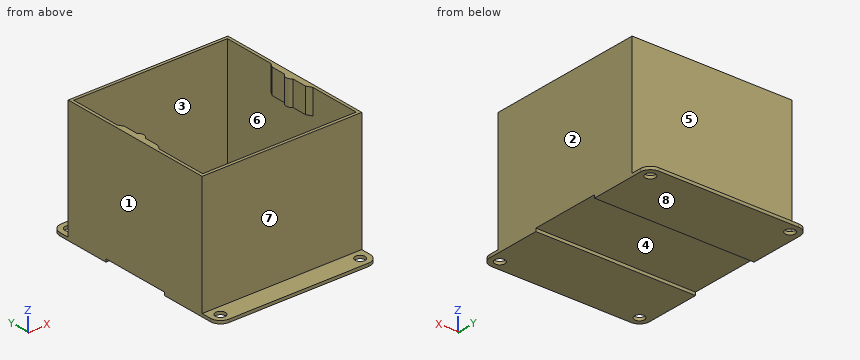
```python
from build123d import *

# Parameters (mm, degrees)
F0_W     = 101.6
F0_H     = 101.6
F1_DEPTH = 76.2
F2_W     = 97.80524
F2_H     = 97.80524
F3_DEPTH = 74.30262
F5_DEPTH = 15.875
F6_R     = 3.175
F7_DEPTH = 1.89738


with BuildPart() as f1:
    # F0 (on Top) → F1 (new body)
    with BuildSketch(Plane.XY):
        Rectangle(F0_W, F0_H)
    extrude(amount=F1_DEPTH)

    # F2 (on face) → F3 (cut)
    with BuildSketch(Plane.XY.offset(76.2)):
        Rectangle(F2_W, F2_H)
    extrude(amount=-F3_DEPTH, mode=Mode.SUBTRACT)

    # F4 (on face) → F5 (join)
    with BuildSketch(Plane.XY.offset(76.2)):
        with BuildLine():
            Line((-47.00524, 12.7), (-48.90262, 15.986359))
            Line((-48.90262, 15.986359), (-48.90262, -15.986359))
            Line((-48.90262, -15.986359), (-47.00524, -12.7))
            Line((-47.00524, -12.7), (-47.00524, -3.175))
            ThreePointArc((-47.00524, -3.175), (-45.301297, 0), (-47.00524, 3.175))
            Line((-47.00524, 3.175), (-47.00524, 12.7))
        make_face()
        with BuildLine():
            Line((48.90262, -15.986359), (48.90262, 15.986359))
            Line((48.90262, 15.986359), (47.00524, 12.7))
            Line((47.00524, 12.7), (47.00524, 3.175))
            ThreePointArc((47.00524, 3.175), (45.301297, 0), (47.00524, -3.175))
            Line((47.00524, -3.175), (47.00524, -12.7))
            Line((47.00524, -12.7), (48.90262, -15.986359))
        make_face()
    extrude(amount=-F5_DEPTH)

    # F6 (on face) → F7 (join)
    with BuildSketch(Plane(origin=(0, 0, 0), x_dir=(1, 0, 0), z_dir=(0, 0, -1))):
        with BuildLine():
            Line((-50.8, 57.15), (-50.8, 22.225))
            Line((-50.8, 22.225), (50.8, 22.225))
            Line((50.8, 22.225), (50.8, 57.15))
            ThreePointArc((50.8, 57.15), (48.940128, 61.640128), (44.45, 63.5))
            Line((44.45, 63.5), (-44.45, 63.5))
            ThreePointArc((-44.45, 63.5), (-48.940128, 61.640128), (-50.8, 57.15))
        make_face()
        with Locations((-44.45, 57.15)):
            Circle(F6_R, mode=Mode.SUBTRACT)
        with Locations((44.45, 57.15)):
            Circle(F6_R, mode=Mode.SUBTRACT)
        with BuildLine():
            Line((50.8, -22.225), (-50.8, -22.225))
            Line((-50.8, -22.225), (-50.8, -57.15))
            ThreePointArc((-50.8, -57.15), (-48.940128, -61.640128), (-44.45, -63.5))
            Line((-44.45, -63.5), (44.45, -63.5))
            ThreePointArc((44.45, -63.5), (48.940128, -61.640128), (50.8, -57.15))
            Line((50.8, -57.15), (50.8, -22.225))
        make_face()
        with Locations((-44.45, -57.15)):
            Circle(F6_R, mode=Mode.SUBTRACT)
        with Locations((44.45, -57.15)):
            Circle(F6_R, mode=Mode.SUBTRACT)
    extrude(amount=F7_DEPTH)


solid = f1.part
```
Read the model definition and answer for the solid it produces. Units are mm, in the model's axes. Face numbers are marked on the shaded views. A direction names the side the tool comes from. Coordinates: 2 decimals unless noted, no trailing zeros. Loops run counter-clockwise (first coordinate to the right, second up) from the corner with the lowest first, then second, coordinate; pieces in that order, holes last. Notation, with made-up numbers: (1.25, 67) -> (21.25, 67) arc R23 ccw to (21.25, 101) -> close; hole circle Ø1 at (-12, 37). An arc over 180 degrees is marked (long way). Return JSON: item names as keys, results as strings.
Item 1: For a pull along X with two mould halves and no side action, classify the marked faces 1, 2, 3 and 4 as +X half, -X half, draft (parallel to the pull), parting line (faces both ways), or undercut.
Answers:
{"face 1": "-X half", "face 2": "+X half", "face 3": "undercut", "face 4": "draft"}
Item 2: Find section C-C (x = 18). Determine the outline of the cut face in (y, z) (3 decimals), plus the area to 3 significant figures.
Answers:
{"outline": "(-63.5, -1.897) -> (-22.225, -1.897) -> (-22.225, 0) -> (22.225, 0) -> (22.225, -1.897) -> (63.5, -1.897) -> (63.5, 0) -> (50.8, 0) -> (50.8, 76.2) -> (48.903, 76.2) -> (48.903, 1.897) -> (-48.903, 1.897) -> (-48.903, 76.2) -> (-50.8, 76.2) -> (-50.8, 0) -> (-63.5, 0) -> close", "area": "631 mm2"}
Item 3: Find section A-A (z = 67). Determine the outline of the cut face in (x, y) (3 decimals), plus the area to 3 significant figures.
Answers:
{"outline": "(-50.8, -50.8) -> (50.8, -50.8) -> (50.8, 50.8) -> (-50.8, 50.8) -> close; hole (-48.903, -48.903) -> (48.903, -48.903) -> (48.903, -15.986) -> (47.005, -12.7) -> (47.005, -3.175) arc R3.81 cw to (47.005, 3.175) -> (47.005, 12.7) -> (48.903, 15.986) -> (48.903, 48.903) -> (-48.903, 48.903) -> (-48.903, 15.986) -> (-47.005, 12.7) -> (-47.005, 3.175) arc R3.81 cw to (-47.005, -3.175) -> (-47.005, -12.7) -> (-48.903, -15.986) -> close", "area": "881 mm2"}
Item 4: Flat-ended cylindrical pins translate along their axes: P1, Ø4, axis at x = -44.45, y = -57.15, coming from the -Z side; P2, Ø1, axis at x = 12, z = 36.5, coming from the -Y side; P3, Ø8.5, axis at x = -44.45, y = 57.15, coming from the +Z side; P4, Ø4, axis at x = -46.5, y = 4, coming from the -Z side. Find the tip coordinate at first contact, or state that the pin passes through.
Answers:
{"P1": "passes through", "P2": "stops at y = -50.8", "P3": "stops at z = 0", "P4": "stops at z = 0"}
Item 5: Find the intervals of material crossed by probe 1 along X at (y, z) = (57.15, -0.8) (3 decimals); probe 2 along Y at (x, z) = (44.45, -0.5) (3 decimals); probe 3 along Y at (x, z) = (44.5, 62.5), in increasing order.
Answers:
{"probe 1": "x = -50.8 to -47.625, -41.275 to 41.275, 47.625 to 50.8", "probe 2": "y = -63.5 to -60.325, -53.975 to -22.225, 22.225 to 53.975, 60.325 to 63.5", "probe 3": "y = -50.8 to -48.9, 48.9 to 50.8"}
Item 6: For the marked faces 5, 6, 7 and 8, determine the directions among +Z, -Z, +X, -X, +Y, -Y from which every point of the face is accessible in a straight line to the end or side of a thin tool.
Answers:
{"face 5": "+Z, +X, -X, +Y", "face 6": "none", "face 7": "+Z, +X, -X, -Y", "face 8": "-Z, +X, -X, +Y, -Y"}
Item 7: Find section B-B (y = -39). Determine the outline of the cut face in (x, z).
Answers:
{"outline": "(-50.8, -1.9) -> (50.8, -1.9) -> (50.8, 76.2) -> (48.9, 76.2) -> (48.9, 1.9) -> (-48.9, 1.9) -> (-48.9, 76.2) -> (-50.8, 76.2) -> close"}
Item 8: Find section D-D (y = 55.5). Determine the outline of the cut face in (x, z), plus the area to 3 significant figures.
Answers:
{"outline": "(-50.8, -1.9) -> (-47.16, -1.9) -> (-47.16, 0) -> (-50.8, 0) -> close; (-41.74, -1.9) -> (41.74, -1.9) -> (41.74, 0) -> (-41.74, 0) -> close; (47.16, -1.9) -> (50.8, -1.9) -> (50.8, 0) -> (47.16, 0) -> close", "area": "172 mm2"}
